Here's how the part is built. I have some questions about the finished solid (model axes, mm). A direction names the side the tool comes from. Coordinates: 2 decimals unless noted, no trailing zeros. Write each loop counter-clockwise with the first axis right and the second up, starting at its lowest first coordinate (ties: lowest second). Pieces come first, ordered by that corner, then holes. Notation, with made-up numbers: (-34, 41) -> (-17, 41) arc R14 cw to (-17, 55) -> close; hole circle Ø1 at (76.25, 80.5). An arc over 180 degrees is marked (long way). Put each result on its own line as item: value. Start each with the question number.
Item 1: If we mould it in two halves opening along X, with no side actions, what happens to faces 3 (the face through (0, -7, 1)), 4 (the face through (15, -13, 20)), 5 (the face through (-4.519, -13.768, 13.617))? For each: released by +X, released by -X, zero draft, split by the parting line, or undercut.
Item 2: For pin 1 (6 mm diameter, centred on x = -8, z = 7.5, fed in from +Y); pin 2 (4.5 mm diameter, centred on x = 11, y = -9.8, fed in from +Z), each with a flat end and sliding along its axis, tell me the tip position at first contact or that it passes through.
Item 3: I want a section at D-D, the plane y = -11.75. List the corners of the cut face in (x, z) for me, then the cut area to 3 significant figures.
Item 4: I want a section at B-B, the plane y = -9.8. List the corners of the cut face in (x, z) for me, then the cut area to 3 significant figures.
Item 5: I need wall thicknesses on line 1 (X direction, y = -9.8, z = 38.05); line 2 (Z direction, x = 6.5, y = -7.25); line 3 (Y direction, x = -11.5, z = 17). Which ranges of each line are inside material? Lowest first, please. Write a range as [from, to].
Item 6: I want a section at C-C, the plane z = 18. List the corners of the cut face in (x, y) for me.
Item 7: I want a section at A-A, the plane x = 8. List the corners of the cut face in (y, z) for me.
Item 8: On a 3-axis mill with a long thin cutter (end or side, diameter ignored), from which of +Z, -Z, +X, -X, +Y, -Y can I reach the whole of each face in a straight line? I mean faces 1 (the face through (0, -7, 39)), 2 (the face through (0, -9, 37.5)). Say none if no direction works.
from build123d import *

# Parameters (mm, degrees)
ESBO_O1_W                = 30
ESBO_O1_H                = 30
RESSALTO_EXTRUS_O1_DEPTH = 40
ESBO_O2_W                = 35
ESBO_O2_H                = 27.5
CORTE_EXTRUS_O1_DEPTH    = 40
FILETE1_R                = 2
FILETE2_R                = 2
ESBO_O4_R                = 5
CORTE_EXTRUS_O3_DEPTH    = 53.201532545
ESBO_O5_R                = 1.35
CORTE_EXTRUS_O5_DEPTH    = 53.201532545
ESBO_O7_R                = 1.35
CORTE_EXTRUS_O6_DEPTH    = 46.276925691
ESBO_O8_W                = 30
ESBO_O8_H                = 22
CORTE_EXTRUS_O8_DEPTH    = 46.276925691
FILETE3_R                = 2
ESBO_O10_R               = 1.35
CORTE_EXTRUS_O9_DEPTH    = 46.276925691


with BuildPart() as part:
    # Esboço1 → Ressalto-extrusão1 (new body)
    with BuildSketch(Plane.XY):
        Rectangle(ESBO_O1_W, ESBO_O1_H)
    extrude(amount=RESSALTO_EXTRUS_O1_DEPTH)

    # Esboço2 → Corte-extrusão1 (cut)
    with BuildSketch(Plane(origin=(15, 0, 0), x_dir=(0, 0, -1), z_dir=(1, 0, 0))):
        with Locations((-20, 1.25)):
            Rectangle(ESBO_O2_W, ESBO_O2_H)
    extrude(amount=-CORTE_EXTRUS_O1_DEPTH, mode=Mode.SUBTRACT)

    # Filete1
    filete1_edges = [part.edges().sort_by_distance(p)[0] for p in [
        (-15, 15, 1.25),
        (15, 15, 1.25),
        (-15, 15, 38.75),
        (15, 15, 38.75),
    ]]
    fillet(filete1_edges, radius=FILETE1_R)

    # Filete2
    filete2_edges = [part.edges().sort_by_distance(p)[0] for p in [
        (0, -15, 40),
        (0, -12.5, 2.5),
        (0, -12.5, 37.5),
        (0, -15, 0),
    ]]
    fillet(filete2_edges, radius=FILETE2_R)

    # Esboço4 → Corte-extrusão3 (cut, through all)
    with BuildSketch(Plane(origin=(0, -15, 0), x_dir=(-1, 0, 0), z_dir=(0, -1, 0))):
        with Locations(Location((0, -20, 0), (0, 0, 90))):
            Circle(ESBO_O4_R)
    extrude(amount=-CORTE_EXTRUS_O3_DEPTH, mode=Mode.SUBTRACT)

    # Esboço5 → Corte-extrusão5 (cut, through all)
    with BuildSketch(Plane(origin=(0, -15, 0), x_dir=(-1, 0, 0), z_dir=(0, -1, 0))):
        with Locations(Location((0, -28, 0), (0, 0, 90))):
            Circle(ESBO_O5_R)
        with Locations(Location((-5.656854249, -25.656854249, 0), (0, 0, 90))):
            Circle(ESBO_O5_R)
        with Locations(Location((-8, -20, 0), (0, 0, 90))):
            Circle(ESBO_O5_R)
        with Locations(Location((-5.656854251, -14.343145752, 0), (0, 0, 90))):
            Circle(ESBO_O5_R)
        with Locations(Location((0, -12, 0), (0, 0, 90))):
            Circle(ESBO_O5_R)
        with Locations(Location((5.656854251, -14.343145752, 0), (0, 0, 90))):
            Circle(ESBO_O5_R)
        with Locations(Location((8, -20, 0), (0, 0, 90))):
            Circle(ESBO_O5_R)
        with Locations(Location((5.656854249, -25.656854249, 0), (0, 0, 90))):
            Circle(ESBO_O5_R)
    extrude(amount=-CORTE_EXTRUS_O5_DEPTH, mode=Mode.SUBTRACT)

    # Esboço7 → Corte-extrusão6 (cut, through all)
    with BuildSketch(Plane(origin=(0, 0, 0), x_dir=(-1, 0, 0), z_dir=(0, 0, -1))):
        with Locations((-11, 12.2)):
            Circle(ESBO_O7_R)
        with Locations((11, 12.2)):
            Circle(ESBO_O7_R)
    extrude(amount=-CORTE_EXTRUS_O6_DEPTH, mode=Mode.SUBTRACT)

    # Esboço8 → Corte-extrusão8 (cut, through all)
    with BuildSketch(Plane(origin=(0, 0, 0), x_dir=(-1, 0, 0), z_dir=(0, 0, -1))):
        with Locations((0, 4)):
            Rectangle(ESBO_O8_W, ESBO_O8_H)
    extrude(amount=-CORTE_EXTRUS_O8_DEPTH, mode=Mode.SUBTRACT)

    # Filete3
    filete3_edges = [part.edges().sort_by_distance(p)[0] for p in [
        (-15, -7, 38.75),
        (-15, -7, 1.25),
        (15, -7, 38.75),
        (15, -7, 1.25),
    ]]
    fillet(filete3_edges, radius=FILETE3_R)

    # Esboço10 → Corte-extrusão9 (cut, through all)
    with BuildSketch(Plane(origin=(0, 0, 0), x_dir=(-1, 0, 0), z_dir=(0, 0, -1))):
        with Locations((-11, -9.8)):
            Circle(ESBO_O10_R)
        with Locations((11, -9.8)):
            Circle(ESBO_O10_R)
    extrude(amount=-CORTE_EXTRUS_O9_DEPTH, mode=Mode.SUBTRACT)


solid = part.part
Calculated:
1. face 3: zero draft
1. face 4: released by +X
1. face 5: undercut
2. pin 1: stops at y = -12.5
2. pin 2: stops at z = 40
3. outline: (-15, 0) -> (15, 0) -> (15, 2.94) -> (-15, 2.94) -> close; (-15, 37.06) -> (15, 37.06) -> (15, 40) -> (-15, 40) -> close
3. area: 176 mm2
4. outline: (-15, 0) -> (-12.35, 0) -> (-12.35, 2.5) -> (-15, 2.5) -> close; (-15, 37.5) -> (-12.35, 37.5) -> (-12.35, 40) -> (-15, 40) -> close; (-9.65, 0) -> (9.65, 0) -> (9.65, 2.5) -> (-9.65, 2.5) -> close; (-9.65, 37.5) -> (9.65, 37.5) -> (9.65, 40) -> (-9.65, 40) -> close; (12.35, 0) -> (15, 0) -> (15, 2.5) -> (12.35, 2.5) -> close; (12.35, 37.5) -> (15, 37.5) -> (15, 40) -> (12.35, 40) -> close
4. area: 123 mm2
5. line 1: x = [-15, -12.35], [-9.65, 9.65], [12.35, 15]
5. line 2: z = [0, 2.5], [37.5, 40]
5. line 3: y = [-15, -12.5]
6. outline: (-15, -15) -> (-4.58, -15) -> (-4.58, -12.5) -> (-15, -12.5) -> close; (4.58, -15) -> (15, -15) -> (15, -12.5) -> (4.58, -12.5) -> close
7. outline: (-15, 2) arc R2 ccw to (-13, 0) -> (-7, 0) -> (-7, 2.5) -> (-10.5, 2.5) arc R2 cw to (-12.5, 4.5) -> (-12.5, 18.65) -> (-15, 18.65) -> close; (-15, 21.35) -> (-12.5, 21.35) -> (-12.5, 35.5) arc R2 cw to (-10.5, 37.5) -> (-7, 37.5) -> (-7, 40) -> (-13, 40) arc R2 ccw to (-15, 38) -> close
8. face 1: +Z, -Z, +X, -X, +Y
8. face 2: +X, -X, +Y
